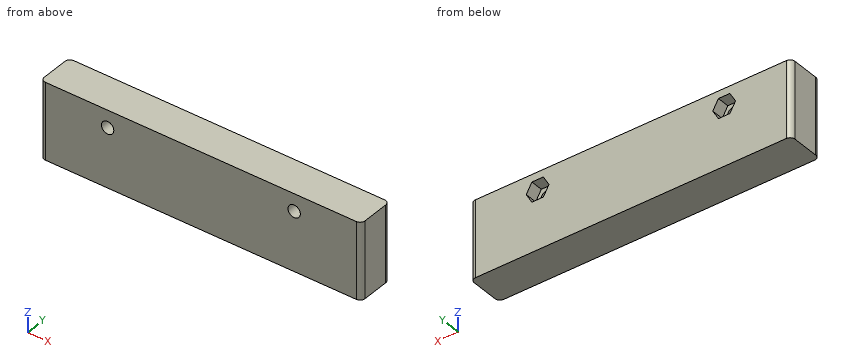
Autodesk Inventor part; units mm, degrees
ref_plane "YZ Plane" through (0, 0, 0) normal (1, 0, 0) x (0, 1, 0)
ref_plane "XZ Plane" through (0, 0, 0) normal (0, 1, 0) x (-1, 0, 0)
ref_plane "XY Plane" through (0, 0, 0) normal (0, 0, 1) x (1, 0, 0)
sketch "Sketch1" plane through (0, 0, 0) normal (0, 0, 1) x (1, 0, 0)
  line L0 (2, 0) -> (128, 0)
  line L1 (130, 2) -> (130, 13)
  line L2 (128, 15) -> (2, 15)
  line L3 (0, 13) -> (0, 2)
  arc A0 (130, 13) -> (128, 15) centre (128, 13) ccw
  arc A1 (128, 0) -> (130, 2) centre (128, 2) ccw
  arc A2 (0, 2) -> (2, 0) centre (2, 2) ccw
  arc A3 (2, 15) -> (0, 13) centre (2, 13) ccw
  point P0 (0, 0)
  point P1 (130, 15)
  point P2 (130, 0)
  point P3 (0, 15)
  dimension "d0" = 130
  dimension "d1" = 15
  dimension "d2" = 2
extrude "Extrusion1" add sketch "Sketch1" along normal blind 31
sketch "Sketch4" plane through (2, 15, 0) normal (0, 1, 0) x (1, 0, 0)
  circle A0 centre (100.8, -24) radius 2.5
  circle A1 centre (25.2, -24) radius 2.5
  line L0 (0, 0) -> (126, 0)
  line L1 (126, -31) -> (0, -31)
  point P0 (-2, 0)
  dimension "d31" = 5
  dimension "d32" = 100.8
  dimension "d33" = 126
  dimension "d34" = 25.2
  dimension "d35" = 24
  dimension "d36" = 24
  dimension "d42" = 7
extrude "Extrusion5" cut sketch "Sketch4" against normal up to next
sketch "Sketch5" plane through (2, 15, 0) normal (0, 1, 0) x (1, 0, 0)
  circle A0 centre (100.8, -24) radius 2.5
  circle A1 centre (25.2, -24) radius 2.5
  line L0 (98.4906, -20) -> (103.1094, -20)
  line L1 (103.1094, -20) -> (105.4188, -24)
  line L2 (105.4188, -24) -> (103.1094, -28)
  line L3 (103.1094, -28) -> (98.4906, -28)
  line L4 (98.4906, -28) -> (96.1812, -24)
  line L5 (96.1812, -24) -> (98.4906, -20)
  line L6 (22.8906, -20) -> (27.5094, -20)
  line L7 (27.5094, -20) -> (29.8188, -24)
  line L8 (29.8188, -24) -> (27.5094, -28)
  line L9 (27.5094, -28) -> (22.8906, -28)
  line L10 (22.8906, -28) -> (20.5812, -24)
  line L11 (20.5812, -24) -> (22.8906, -20)
  point P0 (-2, 0)
  point P1 (25.2, -28)
  point P2 (100.8, -28)
  dimension "d39" = 8
extrude "Extrusion6" cut sketch "Sketch5" against normal blind 5 contours A1 | L0 L1 L2 L3 L4 L5 | L6 L7 L8 L9 L10 L11
equation "\"d32\" = 0.8 * d33"
equation "\"d34\" = 0.2 * d33"
equation "\"d36\" = d35"
properties part number "License_plate_mount"
The model under review builds one solid part; all positions refer to its coordinate system, in mm. Round coordinates to 2 decimals unless told otherwise and drop trailing zeros. Order: outer loops, then holes, each group sorted by start corner. A loop starts at its lowest first (then second) coordinate and runs counter-clockwise, first axis right, second up. Notation, with made-up numbers: (0.5, 49.25) - (23.5, 49.25) arc R17 cw to (23.5, 56.25) - close; hole circle Ø11 at (-23, 56.5). An arc over 180 degrees is marked (long way). Answer in a Markdown table with one row per item.
(1) Clearance check with flat-ended pins moving along their axes: P1, Ø2.5, axis at x = 104.5, z = 23, coming from the +Y side; P2, Ø4.5, axis at x = 27.2, z = 24, coming from the +Y side. State where each tip first meets the part, or that it passes through.
Result set:
| item | result |
|---|---|
| P1 | stops at y = 10 |
| P2 | passes through |
(2) For line 1 (X direction, y = 3, z = 24); line 2 (Z direction, x = 102.8, y = 3); line 3 (Z direction, x = 101, y = 14.25), list the stretches that pass through material, from the lowest coordinate up. Write a range as from..to.
Result set:
| item | result |
|---|---|
| line 1 | x = 0..24.7, 29.7..100.3, 105.3..130 |
| line 2 | z = 0..21.5, 26.5..31 |
| line 3 | z = 0..20, 28..31 |
(3) Take a section at A-A on x = 27.2. Write out the cut boundary in (y, z), plus the area to 3 significant figures.
Result set:
| item | result |
|---|---|
| outline | (0, 0) - (15, 0) - (15, 20) - (10, 20) - (10, 21.5) - (0, 21.5) - close; (0, 26.5) - (10, 26.5) - (10, 28) - (15, 28) - (15, 31) - (0, 31) - close |
| area | 375 mm2 |
